```python
from build123d import *

# Parameters (mm, degrees)
EXTRUDE_1_DEPTH     = 29
SKETCH_2_R          = 2.25
CUT_EXTRUDE_1_DEPTH = 90
SKETCH_3_R          = 2.25
CUT_EXTRUDE_2_DEPTH = 40


with BuildPart() as part:
    # 草图1 → 凸台-拉伸1 (new body)
    with BuildSketch(Plane(origin=(0, 0, 0), x_dir=(0, 0, -1), z_dir=(1, 0, 0))):
        with BuildLine():
            Line((0, 0), (350, 0))
            ThreePointArc((350, 0), (366, 16), (350, 32))
            Line((350, 32), (150, 32))
            Line((150, 32), (150, 56))
            Line((150, 56), (350, 56))
            ThreePointArc((350, 56), (390, 16), (350, -24))
            Line((350, -24), (0, -24))
            Line((0, -24), (0, 0))
        make_face()
    extrude(amount=EXTRUDE_1_DEPTH)

    # 草图2 → 切除-拉伸1 (cut)
    with BuildSketch(Plane(origin=(0, 0, 0), x_dir=(1, 0, 0), z_dir=(0, 1, 0))):
        with Locations((36, 15)):
            Circle(SKETCH_2_R)
        with Locations(Location((11, 15, 0), (0, 0, 270))):
            Circle(SKETCH_2_R)
    extrude(amount=-CUT_EXTRUDE_1_DEPTH, mode=Mode.SUBTRACT)

    # 草图3 → 切除-拉伸2 (cut)
    with BuildSketch(Plane(origin=(0, 56, 0), x_dir=(1, 0, 0), z_dir=(0, 1, 0))):
        with Locations(Location((11, 165, 0), (0, 0, 270))):
            Circle(SKETCH_3_R)
        with Locations((36, 165)):
            Circle(SKETCH_3_R)
    extrude(amount=-CUT_EXTRUDE_2_DEPTH, mode=Mode.SUBTRACT)


solid = part.part
```
For this review, take the finished solid that the model builds, in its own axes (mm). A direction names the side the tool comes from. Coordinates: 2 decimals unless noted, no trailing zeros. Loops run counter-clockwise (first coordinate to the right, second up) from the corner with the lowest first, then second, coordinate; pieces in that order, holes last. Notation, with made-up numbers: (58, 39) -> (100, 39) arc R26 ccw to (100, 56) -> close; hole circle Ø4 at (66.5, 49.25). An arc over 180 degrees is marked (long way). Return JSON: item names as keys, results as strings. Group by question number.
(1) Consider section C-C, the plane y = -7. Give the boundary of the cut face in (x, z).
(2) Consider section D-D, the plane z = -75. Give the boundary of the cut face in (x, y).
(3) Tool access review of faces 1 (the flat face through (14, 44, -150)), 2 (the cylindrical face through (14, 16, -366)): name each direction out of +Z, -Z, +X, -X, +Y, -Y from which nothing blocks a thin tool from reaching the whole face with its end or side.
(4) Consider section A-A, the plane x = 24.75. Give the boundary of the cut face in (y, z), plus the area to 3 significant figures.
(5) For pin 1 Ø1 at (x, y) = (4.5, 47.5) entering from -Z; pin 2 Ø2.5 at (x, z) = (11, -165) entering from +Y; pin 3 Ø8 at (y, z) = (38.5, -264.5) entering from -X; pin 4 Ø12 at (x, y) = (15, 40) entering from +Z, all flat-tipped, find the tip position at first contact; note any pin that passes through.
(6) To check wall thickness, follow L1, parallel to X at y = 45.25, z = -165; L2, parallel to Y at x = 27, z = -151.5; L3, parallel to Y at x = 10.75, z = -37. State the ranges of each line that lie inside material, in increasing order.
(7) Mouldability with a two-part tool opening along Y and no side actions: class faces 3 (the flat face through (14, 32, -251)), 4 (the flat face through (14, 56, -249)), 5 (the flat face through (14, 0, -173)), 6 (the flat face through (14, -12, 0)) as pulls with the +Y half, pulls with the -Y half, needs draft (parallel to the pull), parting line crosses it, or undercut.
(8) Consider section B-B, the plane z = -332. Give the boundary of the cut face in (x, y), plus the area to 3 significant figures.
Results below:
{
 "1": {"outline": "(0, -382.73) -> (29, -382.73) -> (29, 0) -> (0, 0) -> close; hole circle Ø4.5 at (11, -15)"},
 "2": {"outline": "(0, -24) -> (29, -24) -> (29, 0) -> (0, 0) -> close"},
 "3": {"face 1": "+Z, +X, -X, +Y", "face 2": "+Z, +X, -X"},
 "4": {"outline": "(-24, -350) arc R40 ccw to (56, -350) -> (56, -150) -> (32, -150) -> (32, -350) arc R16 cw to (0, -350) -> (0, 0) -> (-24, 0) -> close", "area": "15,300 mm2"},
 "5": {"pin 1": "stops at z = -375.28", "pin 2": "stops at y = 0", "pin 3": "stops at x = 0", "pin 4": "stops at z = -150"},
 "6": {"L1": "x = 0 to 8.75, 13.25 to 29", "L2": "y = -24 to 0, 32 to 56", "L3": "y = -24 to 0"},
 "7": {"face 3": "undercut", "face 4": "pulls with the +Y half", "face 5": "undercut", "face 6": "needs draft"},
 "8": {"outline": "(0, -24) -> (29, -24) -> (29, 0) -> (0, 0) -> close; (0, 32) -> (29, 32) -> (29, 56) -> (0, 56) -> close", "area": "1,390 mm2"}
}
